from build123d import *

# Parameters (mm, degrees)
SKETCH1_R           = 2.413
BOSS_EXTRUDE1_DEPTH = 25.4
SKETCH2_R           = 3.96875
BOSS_EXTRUDE2_DEPTH = 4.826
CUT_EXTRUDE1_DEPTH  = 3.81


with BuildPart() as part:
    # Sketch1 → Boss-Extrude1 (new body)
    with BuildSketch(Plane.XY):
        Circle(SKETCH1_R)
    extrude(amount=BOSS_EXTRUDE1_DEPTH)

    # Sketch2 → Boss-Extrude2 (add)
    with BuildSketch(Plane.XY.offset(25.4)):
        Circle(SKETCH2_R)
    extrude(amount=BOSS_EXTRUDE2_DEPTH)

    # Sketch3 → Cut-Extrude1 (cut)
    with BuildSketch(Plane.XY.offset(30.226)):
        Polygon((2.291358881, 0), (1.14567944, 1.984375), (-1.14567944, 1.984375), (-2.291358881, 0), (-1.14567944, -1.984375), (1.14567944, -1.984375), align=None)
    extrude(amount=-CUT_EXTRUDE1_DEPTH, mode=Mode.SUBTRACT)


solid = part.part
The listing builds one solid part. Answer for the finished solid, in the listing's coordinates (mm). A direction names the side the tool comes from. Coordinates: 2 decimals unless noted, no trailing zeros. Loops run counter-clockwise (first coordinate to the right, second up) from the corner with the lowest first, then second, coordinate; pieces in that order, holes last.
1) Determine the mould class of faces 4 (the face through (0, 1.984, 28)), 5 (the face through (-0.86, -3.874, 27.779)), 6 (the face through (-2, -1, 30.226)), 7 (the face through (-1.727, -0.978, 28.348)) for opening direction Y: pulls with the +Y half, pulls with the -Y half, needs draft (parallel to the pull), parting line crosses it, or undercut.
2) Flat-ended cylindrical pins translate along their axes: pin 1 Ø4.5 at (x, y) = (-1, 0.5) entering from +Z; pin 2 Ø3 at (y, z) = (0, 20) entering from -X; pin 3 Ø1.5 at (x, z) = (-1.5, 10) entering from +Y; pin 4 Ø1 at (y, z) = (2.5, 25) entering from -X. Find the tip coordinate at first contact, or state that the pin passes through.
3) Find the intervals of material crossed by L1, parallel to Z at x = 2, y = 3.25; L2, parallel to Y at x = 0, z = 17; L3, parallel to X at y = 0.75, z = 5.5, in increasing order.
4) Find section A-A on z = 28. Write down the section's boundary in (x, y), then the cut area to 3 significant figures.
5) Find section B-B on x = 0. Write down the section's boundary in (y, z), then the cut area to 3 significant figures.
6) A tool of negligible diameter and unlimited length cuts with its end or side. For faces 1 (the face through (-1.71, 1.01, 28.35)), 2 (the face through (0, 0, 0)), 3 (the face through (2, -2, 25.4)), from which of +Z, -Z, +X, -X, +Y, -Y can it reach the whole face along a straight path? Write none if from no direction.
7) Find section C-C on z = 22.5. Write down the section's boundary in (x, y).
Values:
1. face 4: undercut
1. face 5: parting line crosses it
1. face 6: needs draft
1. face 7: undercut
2. pin 1: stops at z = 30.23
2. pin 2: stops at x = -2.41
2. pin 3: stops at y = 2.29
2. pin 4: stops at x = -3.3
3. L1: z = 25.4 to 30.23
3. L2: y = -2.41 to 2.41
3. L3: x = -2.29 to 2.29
4. outline: circle Ø7.94 at (0, 0); hole (-2.29, 0) - (-1.15, -1.98) - (1.15, -1.98) - (2.29, 0) - (1.15, 1.98) - (-1.15, 1.98) - close
4. area: 35.8 mm2
5. outline: (-3.97, 25.4) - (-2.41, 25.4) - (-2.41, 0) - (2.41, 0) - (2.41, 25.4) - (3.97, 25.4) - (3.97, 30.23) - (1.98, 30.23) - (1.98, 26.42) - (-1.98, 26.42) - (-1.98, 30.23) - (-3.97, 30.23) - close
5. area: 146 mm2
6. face 1: +Z
6. face 2: -Z, +X, -X, +Y, -Y
6. face 3: -Z
7. outline: circle Ø4.83 at (0, 0)
